from build123d import *

# Parameters (mm, degrees)
BOSS_EXTRUDE1_DEPTH = 41.2
SKETCH4_W           = 36.8
SKETCH4_H           = 61.2
CUT_EXTRUDE1_DEPTH  = 10000
SKETCH5_R           = 10
BOSS_EXTRUDE2_DEPTH = 5
FILLET1_R           = 12.5


with BuildPart() as part:
    # Sketch2 → Boss-Extrude1 (new body)
    with BuildSketch(Plane(origin=(0, 0, 0), x_dir=(0, 0, -1), z_dir=(1, 0, 0))):
        Polygon((0, 0), (-25, 0), (-25, 42.867109497), (-37.3, 61.2), (-37.3, 63.4), (0, 63.4), align=None)
    extrude(amount=BOSS_EXTRUDE1_DEPTH)

    # Sketch4 → Cut-Extrude1 (cut)
    with BuildSketch(Plane.XY):
        with Locations((20.6, 30.6)):
            Rectangle(SKETCH4_W, SKETCH4_H)
    extrude(amount=CUT_EXTRUDE1_DEPTH, mode=Mode.SUBTRACT)

    # Sketch5 → Boss-Extrude2 (add)
    with BuildSketch(Plane(origin=(2.2, 0, 0), x_dir=(0, 0, -1), z_dir=(1, 0, 0))):
        with Locations(Location((-12.5, 12.5, 0), (0, 0, 90))):
            Circle(SKETCH5_R)
    boss_extrude2 = extrude(amount=BOSS_EXTRUDE2_DEPTH)

    # Mirror1: Boss-Extrude2 across plane
    add(boss_extrude2.mirror(Plane(origin=(20.6, 0, 0), x_dir=(0, 0, 1), z_dir=(1, 0, 0))))

    # Fillet1
    fillet1_edges = [part.edges().sort_by_distance(p)[0] for p in [
        (1.1, 0, 25),
        (1.1, 0, 0),
        (40.1, 0, 0),
        (40.1, 0, 25),
    ]]
    fillet(fillet1_edges, radius=FILLET1_R - 0.0001)  # a hair under: the kernel refuses the full size


solid = part.part
Build history of the part. All positions in model axes, mm. A direction names the side the tool comes from. Coordinates: 2 decimals unless noted, no trailing zeros. Order: outer loops, then holes, each group sorted by start corner. A loop starts at its lowest first (then second) coordinate and runs counter-clockwise, first axis right, second up. Notation, with made-up numbers: M 56.25,63.5 L 76.25,63.5 A27 cw 76.25,98.5 Z; hole C -5,-13.5 d10. An arc over 180 degrees is marked long. One line per question, with ' | ' between items. Start each with the question number.
Q1. Flat gauge pins, fed straight in: pin 1 Ø18.5 at (x, z) = (28, 18) entering from -Y; pin 2 Ø2.5 at (x, y) = (40, 29) entering from +Z. Where does each tip first touch, or does it go through?
Q2. Probe L1, parallel to X at y = 55, z = 8; L2, parallel to Y at x = 31, z = 12; L3, parallel to X at y = 9, z = 11.5. List the from-to ranges inside material, lowest first. Write a range as from..to.
Q3. 3-axis set-ups, long thin cutter, end or side, ignore diameter. For faces 1 (the face through (4.665, 17.114, 3.628)), 2 (the face through (2, 46, 0)), 3 (the face through (0, 32, 14)), 4 (the face through (1, 27, 25)), 5 (the face through (7.2, 12, 13)): which of +Z, -Z, +X, -X, +Y, -Y reach the whole face in a straight line?
Q4. Saw through at A-A (y = 47). List the corners of the cut face in (x, z), then the cut area to 3 significant figures.
Q5. Saw through at C-C (z = 20). List the corners of the cut face in (x, y).
Q6. Saw through at B-B (x = 3.5). List the corners of the cut face in (y, z), then the cut area to 3 significant figures.
Q7. Saw through at D-D (y = 15). List the corners of the cut face in (x, z).
Check values:
1) pin 1: stops at y = 2.5 | pin 2: stops at z = 25
2) L1: x = 0..2.2, 39..41.2 | L2: y = 61.2..63.4 | L3: x = 0..7.2, 34..41.2
3) face 1: none | face 2: -Z, +X, -X, +Y, -Y | face 3: +Z, -Z, -X, +Y, -Y | face 4: +Z, +X, -X, -Y | face 5: +Z, -Z, -Y
4) outline: M 0,0 L 2.2,0 L 2.2,27.77 L 0,27.77 Z; M 39,0 L 41.2,0 L 41.2,27.77 L 39,27.77 Z | area: 122 mm2
5) outline: M 0,2.5 L 2.2,2.5 L 2.2,5.89 L 7.2,5.89 L 7.2,19.11 L 2.2,19.11 L 2.2,61.2 L 39,61.2 L 39,19.11 L 34,19.11 L 34,5.89 L 39,5.89 L 39,2.5 L 41.2,2.5 L 41.2,63.4 L 0,63.4 Z
6) outline: C 12.5,12.5 d20; M 61.2,0 L 63.4,0 L 63.4,37.3 L 61.2,37.3 Z | area: 396 mm2
7) outline: M 0,0 L 2.2,0 L 2.2,2.82 L 7.2,2.82 L 7.2,22.18 L 2.2,22.18 L 2.2,25 L 0,25 Z; M 34,2.82 L 39,2.82 L 39,0 L 41.2,0 L 41.2,25 L 39,25 L 39,22.18 L 34,22.18 Z
